Geometry: final body of the model. Coordinates: model frame, mm. A direction names the side the tool comes from. Give positions to 0.01 mm unless a question says otherwise; leave off trailing zeros. Order: outer loops, then holes, each group sorted by start corner. A loop starts at its lowest first (then second) coordinate and runs counter-clockwise, first axis right, second up. Notation, with made-up numbers: (35.5, 12) -> (57.5, 12) arc R15 ccw to (57.5, 21) -> close; hole circle Ø11 at (46.25, -9.75). An arc over 180 degrees is marked (long way). Write item = value, one per line.
```python
from build123d import *

# Parameters (mm, degrees)
SKETCH1_W               = 8
SKETCH1_H               = 8
BOSS_EXTRUDE1_DEPTH     = 3
CUT_EXTRUDE1_DEPTH      = 12.704699911
CUT_EXTRUDE1_DEPTH_BACK = 12.704699911
CUT_EXTRUDE2_DEPTH      = 11
SKETCH4_R               = 1.75
CUT_EXTRUDE3_DEPTH      = 0.4
SKETCH5_W               = 8
SKETCH5_H               = 1
BOSS_EXTRUDE2_DEPTH     = 2
FILLET1_R               = 4
CUT_EXTRUDE4_DEPTH      = 0.4


with BuildPart() as part:
    # Sketch1 → Boss-Extrude1 (new body)
    with BuildSketch(Plane(origin=(0, 0, 0), x_dir=(1, 0, 0), z_dir=(0, 1, 0))):
        with Locations((4, 4)):
            Rectangle(SKETCH1_W, SKETCH1_H)
    extrude(amount=BOSS_EXTRUDE1_DEPTH)

    # Sketch2 → Cut-Extrude1 (cut, two sides: drawn at the far end of the back side and taken through both)
    with BuildSketch(Plane.XY.offset(-CUT_EXTRUDE1_DEPTH_BACK)):
        Polygon((0, 0), (0.6, 3), (0, 3), align=None)
        Polygon((8, 0), (7.4, 3), (8, 3), align=None)
    extrude(amount=CUT_EXTRUDE1_DEPTH + CUT_EXTRUDE1_DEPTH_BACK, mode=Mode.SUBTRACT)

    # Sketch3 → Cut-Extrude2 (cut)
    with BuildSketch(Plane(origin=(0, 0, 0), x_dir=(0, 0, -1), z_dir=(1, 0, 0))):
        Polygon((0, 0), (0.6, 3), (0, 3), align=None)
        Polygon((8, 3), (7.4, 3), (8, 0), align=None)
    extrude(amount=CUT_EXTRUDE2_DEPTH, mode=Mode.SUBTRACT)

    # Sketch4 → Cut-Extrude3 (cut)
    with BuildSketch(Plane.XZ):
        with Locations(Location((4, -3.75, 0), (0, 0, 270))):
            Circle(SKETCH4_R)
    extrude(amount=-CUT_EXTRUDE3_DEPTH, mode=Mode.SUBTRACT)

    # Sketch5 → Boss-Extrude2 (add)
    with BuildSketch(Plane.XZ):
        with Locations((4, -7.5)):
            Rectangle(SKETCH5_W, SKETCH5_H)
    extrude(amount=BOSS_EXTRUDE2_DEPTH)

    # Fillet1
    # the kernel refuses this fillet: 4 mm, written as the material it takes off along each edge
    with BuildSketch(Plane(origin=(8, -2, -16.660254038), x_dir=(0, 1, 0), z_dir=(0, 0, 1)), Plane(origin=(0, -2, 1.660254038), x_dir=(0, 1, 0), z_dir=(0, 0, -1))) as fillet1_piece_1:
        with BuildLine():
            CenterArc((4, 3.464101615), FILLET1_R, 180, 60)
            Line((0, 3.464101615), (-0.08, 3.464101615))
            Line((-0.08, 3.464101615), (-0.08, 0))
            Line((-0.08, 0), (0, -0.08))
            ThreePointArc((0, -0.08), (1, -0.08), (1.96, -0.069282032))
            Line((1.96, -0.069282032), (2, 0))
        make_face()
    extrude(amount=18.320508076, mode=Mode.SUBTRACT)

    # Sketch6 → Cut-Extrude4 (cut)
    with BuildSketch(Plane(origin=(0, 3, 0), x_dir=(1, 0, 0), z_dir=(0, 1, 0))):
        Polygon((2.030290665, 2.010567225), (2.030290665, 6.010567225), (3.331572716, 6.010567225), (4.004649639, 3.28220184), (4.677726562, 6.010567225), (5.979008613, 6.010567225), (5.979008613, 2.010567225), (5.209777844, 2.010567225), (5.184136818, 5.159605686), (4.433335536, 2.010567225), (3.575963742, 2.010567225), (2.82516246, 5.159605686), (2.799521434, 2.010567225), align=None)
    extrude(amount=-CUT_EXTRUDE4_DEPTH, mode=Mode.SUBTRACT)


solid = part.part
```
1) Section query A-A (y = 0.1). Output: boundary loops of the cut face in (x, z), plus the area to 3 significant figures.
Check sheet entries:
outline = (0.02, -7.98) -> (7.98, -7.98) -> (7.98, -0.02) -> (0.02, -0.02) -> close; hole circle Ø3.5 at (4, -3.75)
area = 53.7 mm²
2) Reachability of faces 1 (the face through (2.94, 0.2, -2.36)), 2 (the face through (4, -1, -7)), 3 (the face through (0.3, 1.5, -4.1)) from +Z, -Z, +X, -X, +Y, -Y: full face, straight path, thin tool, end or side. Return the list, or none.
Check sheet entries:
face_1 = -Y
face_2 = +Z, +X, -X, -Y
face_3 = +Z, -Z, -X, +Y
3) First-contact query: P1, Ø1.2, axis at x = 4.5, z = -4, coming from the +Y side; P2, Ø3, axis at y = -1, z = -2.5, coming from the -X side; P3, Ø4, axis at x = 4.5, z = -3, coming from the -Y side; P4, Ø1, axis at x = 5, y = -1, coming from the +Z side. Flat tips, straight axial feed; report the tip coordinate or a pass-through.
Check sheet entries:
P1 = 3
P2 = 0
P3 = 0
P4 = -7
4) Section query B-B (x = 7.25). Output: boundary loops of the cut face in (y, z).
Check sheet entries:
outline = (-0.94, -8) -> (0, -8) -> (3, -7.4) -> (3, -0.6) -> (0, 0) -> (0, -7) -> (-0.94, -7) -> close
5) Line query: line 1 (Y direction, x = 3, z = -6.5); line 2 (Y direction, x = 2.75, z = -4); line 3 (X direction, y = 0.35, z = -3.75). Output: solid intervals per line, ascending. Write a range as from..to.
Check sheet entries:
line_1 = 0..3
line_2 = 0.4..2.6
line_3 = 0.07..2.25, 5.75..7.93
6) Section query C-C (z = -4.25). Output: boundary loops of the cut face in (x, y), plus the area to 3 significant figures.
Check sheet entries:
outline = (0, 0) -> (2.32, 0) -> (2.32, 0.4) -> (5.68, 0.4) -> (5.68, 0) -> (8, 0) -> (7.4, 3) -> (5.98, 3) -> (5.98, 2.6) -> (5.19, 2.6) -> (5.19, 3) -> (4.97, 3) -> (4.97, 2.6) -> (4.24, 2.6) -> (4.24, 3) -> (3.77, 3) -> (3.77, 2.6) -> (3.04, 2.6) -> (3.04, 3) -> (2.82, 3) -> (2.82, 2.6) -> (2.03, 2.6) -> (2.03, 3) -> (0.6, 3) -> close
area = 19.6 mm²
7) Section query D-D (y = 0.85). Output: boundary loops of the cut face in (x, z), plus the area to 3 significant figures.
Check sheet entries:
outline = (0.17, -7.83) -> (7.83, -7.83) -> (7.83, -0.17) -> (0.17, -0.17) -> close
area = 58.7 mm²
8) Mould query, pull axis Z, two halves, no side actions, for faces 4 (the face through (4.5, 2.6, -4)), 5 (the face through (3.9, 1.5, -0.3)), 6 (the face through (7.7, 1.5, -4.1)). Classes: +Z half, -Z half, draft (parallel to the pull), parting line (faces both ways), or undercut.
Check sheet entries:
face_4 = undercut
face_5 = +Z half
face_6 = draft
